from build123d import *

# Parameters (mm, degrees)
F0_W            = 73.4
F0_H            = 73.4
F0_R            = 2.15
F1_DEPTH        = 1.5748
F2_R            = 0.635
F3_DEPTH        = 1.5758
F4_W            = 5
F4_H            = 5
F5_DEPTH        = 0.0508
F5_COPIES_COUNT = 24
F8_R            = 0.74
F9_DEPTH        = 1.5758
F10_R           = 1.038
F11_DEPTH       = 1.5758
F7_R            = 1.016
F12_DEPTH       = 1.524
F13_R           = 0.635
F14_DEPTH       = 1.5758
F15_R           = 0.635
F16_DEPTH       = 1.5758


# Not quite as in the source:
# - a pattern or mirror of a feature is missing from the dataset's text; its kind, count and spacing are read off the source's solid


with BuildPart() as f1:
    # F0 (on Top) → F1 (new body)
    with BuildSketch(Plane.XY):
        Rectangle(F0_W, F0_H)
        with Locations((-32, -32)):
            Circle(F0_R, mode=Mode.SUBTRACT)
        with Locations((32, -32)):
            Circle(F0_R, mode=Mode.SUBTRACT)
        with Locations((-32, 32)):
            Circle(F0_R, mode=Mode.SUBTRACT)
        with Locations((32, 32)):
            Circle(F0_R, mode=Mode.SUBTRACT)
    extrude(amount=F1_DEPTH)

    # F2 (on Top) → F3 (cut, through all)
    with BuildSketch(Plane.XY):
        with Locations((-33.2, -10.4)):
            Circle(F2_R)
        with Locations((-33.2, 10.4)):
            Circle(F2_R)
        with Locations((11.8, -10.4)):
            Circle(F2_R)
        with Locations((11.8, -2.4)):
            Circle(F2_R)
    extrude(amount=F3_DEPTH, mode=Mode.SUBTRACT)

    # F4 (on face) → F5 (join)
    with BuildSketch(Plane(origin=(0, 0, 0), x_dir=(1, 0, 0), z_dir=(0, 0, -1))):
        with Locations((29.53, 0)):
            Rectangle(F4_W, F4_H)
    f5 = extrude(amount=F5_DEPTH)

    # F5_copies: F5 ×24 about axis
    f5_copies_axis = Axis((0, 0, 0), (0, 0, 1))
    for i in range(1, F5_COPIES_COUNT):
        add(f5.rotate(f5_copies_axis, i * 360 / F5_COPIES_COUNT))

    # F8 (on Top) → F9 (cut, through all)
    with BuildSketch(Plane.XY):
        with Locations((-24.97, 35)):
            Circle(F8_R)
        with Locations((-17.35, 35)):
            Circle(F8_R)
    extrude(amount=F9_DEPTH, mode=Mode.SUBTRACT)

    # F10 (on Top) → F11 (cut, through all)
    with BuildSketch(Plane.XY):
        with Locations((-24.6, 28.53)):
            Circle(F10_R)
        with Locations((-24.6, 23.45)):
            Circle(F10_R)
        with Locations((-33, 24.14)):
            Circle(F10_R)
        with Locations((-33, 19.06)):
            Circle(F10_R)
        with Locations((-33, -19.06)):
            Circle(F10_R)
        with Locations((-33, -24.14)):
            Circle(F10_R)
    extrude(amount=F11_DEPTH, mode=Mode.SUBTRACT)

    # F7 (on Top) → F12 (cut)
    with BuildSketch(Plane.XY):
        Circle(F7_R)
    extrude(amount=F12_DEPTH, mode=Mode.SUBTRACT)

    # F13 (on Top) → F14 (cut, through all)
    with BuildSketch(Plane.XY):
        with Locations((12.98, 33.6)):
            Circle(F13_R)
        with Locations((15.52, 33.6)):
            Circle(F13_R)
        with Locations((18.06, 33.6)):
            Circle(F13_R)
        with Locations((20.6, 33.6)):
            Circle(F13_R)
    extrude(amount=F14_DEPTH, mode=Mode.SUBTRACT)

    # F15 (on Top) → F16 (cut, through all)
    with BuildSketch(Plane.XY):
        with Locations((3.22, -17.7)):
            Circle(F15_R)
        with Locations((3.22, -20.24)):
            Circle(F15_R)
        with Locations((5.76, -20.24)):
            Circle(F15_R)
        with Locations((5.76, -17.7)):
            Circle(F15_R)
        with Locations((8.3, -17.7)):
            Circle(F15_R)
        with Locations((8.3, -20.24)):
            Circle(F15_R)
    extrude(amount=F16_DEPTH, mode=Mode.SUBTRACT)


solid = f1.part
Verification items for the finished model (mm, model axes). Give positions to 0.01 mm unless a question says otherwise; leave off trailing zeros. Write each loop counter-clockwise with the first axis right and the second up, starting at its lowest first coordinate (ties: lowest second). Pieces come first, ordered by that corner, then holes. Notation, with made-up numbers: M 40,-33 L 98,-33 A16 ccw 98,-20 Z; hole C -5,75 d1. An arc over 180 degrees is marked long. Put each result on its own line as item: value. Start each with the question number.
1. Section check B-B (y = 7). Record the cut outline in (x, z).
2. Go/stop test with a flat-tipped pin: pin 1 Ø2 at (x, y) = (11.8, -10.4) entering from -Z. Record where the tip stops, or that it passes through.
3. Draft check along Y on faces 1 (the face through (-34.037, 19.106, 0.776)), 2 (the face through (8, 28, -0.051)), 3 (the face through (-1, -36.7, 1)). Enter one of: +Y half, -Y half, draft (parallel to the pull), parting line (faces both ways), or undercut.
4. Section check A-A (z = 0.65). Give the number of separate pieces and of enclosed holes in the cut face, and give its area (3 significant figures).
5. Scan lines: line 1 along Y through (x, z) = (11.8, 0.5) (3 decimals); line 2 along Y through (x, z) = (5.76, 0.9) (3 decimals); line 3 along Y through (x, z) = (0, 0.6). Record each from-to range of solid material in increasing order. Write a range as [from, to].
Answer list:
1. outline: M -36.7,0 L -31.28,0 L -31.28,-0.05 L -26.11,-0.05 L -26.11,0 L 26.11,0 L 26.11,-0.05 L 31.28,-0.05 L 31.28,0 L 36.7,0 L 36.7,1.57 L -36.7,1.57 Z
2. pin 1: z = 0
3. face 1: undercut
3. face 2: draft
3. face 3: -Y half
4. separate pieces: 1
4. enclosed holes: 27
4. area: 5,280 mm2
5. line 1: [-36.7, -11.035], [-9.765, -3.035], [-1.765, 36.7]
5. line 2: [-36.7, -20.875], [-19.605, -18.335], [-17.065, 36.7]
5. line 3: [-36.7, -1.02], [1.02, 36.7]
